Input: dimensioned drawing with shaded views. Units: mm. Origin: part minimum x, y, z. A direction names the side the tool comes from. Coordinates: 2 decimals unless noted, no trailing zeros. Loops run counter-clockwise (first coordinate to the right, second up) from the corner with the lowest first, then second, coordinate; pieces in that order, holes last.
Item 1: Contact query for flat-ended pins moving along their axis: P1, Ø4, axis at x = 198.5, y = 184.5, coming from the +Z side; P2, Ø6, axis at y = 120, z = 552.5, coming from the -X side; P3, Ø6, axis at y = 65, z = 941.5, coming from the +X side. Output: stop coordinate, or through.
Item 2: Section C-C on z = 563.5. Return loops of the section in (x, y), and give its area (3 significant figures).
Item 3: Section B-B on x = 825.5. Return loops of the section in (y, z).
Item 4: Pull-direction query (Z, two-part tool) for the marked faces 4, 5 and 6; classes: released by +Z, released by -Z, zero draft, split by the parting line, or undercut.
Item 5: Section A-A on y = 143. Return loops of the section in (x, z) (1 decimal), and give its area (3 significant figures).
Item 6: Reachability of the marked faces 1, 2 and 3 from +Z, -Z, +X, -X, +Y, -Y: full face, straight path, thin tool, end or side. Return the list, or none.
Item 7: Section D-D on x = 416. Return loops of the section in (y, z).
Item 8: Ray query, line 1 along Z through (x, y) = (825, 111); line 2 along X through (y, z) = (43.5, 372); line 3 along Z through (x, y) = (148, 86). Return the intervals inside material, ascending.
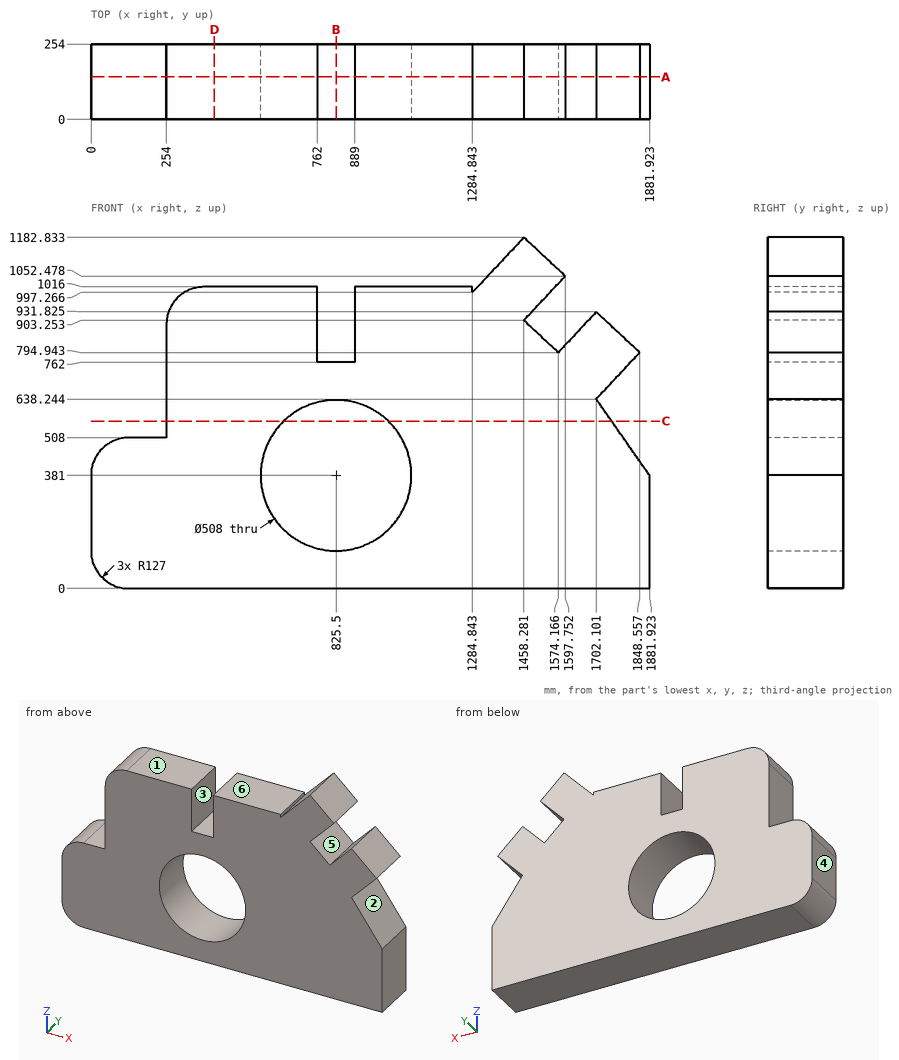
Results found:
1. P1: stops at z = 508
1. P2: stops at x = 254
1. P3: stops at x = 1496.83
2. outline: (254, 0) - (648.84, 0) - (648.84, 254) - (254, 254) - close; (1002.16, 0) - (1754.35, 0) - (1754.35, 254) - (1002.16, 254) - close
2. area: 291,000 mm2
3. outline: (0, 0) - (254, 0) - (254, 127) - (0, 127) - close; (0, 635) - (254, 635) - (254, 762) - (0, 762) - close
4. face 4: zero draft
4. face 5: undercut
4. face 6: released by +Z
5. outline: (0, 127) arc R127 ccw to (127, 0) - (1881.9, 0) - (1881.9, 381) - (1702.1, 638.2) - (1848.6, 794.9) - (1702.1, 931.8) - (1574.2, 794.9) - (1458.3, 903.3) - (1597.8, 1052.5) - (1458.3, 1182.8) - (1284.8, 997.3) - (1284.8, 1016) - (889, 1016) - (889, 762) - (762, 762) - (762, 1016) - (381, 1016) arc R127 ccw to (254, 889) - (254, 508) - (127, 508) arc R127 ccw to (0, 381) - close; hole circle Ø508 at (825.5, 381)
5. area: 1,460,000 mm2
6. face 1: +Z, -X, +Y, -Y
6. face 2: +X, +Y, -Y
6. face 3: +Z, +Y, -Y
7. outline: (0, 0) - (254, 0) - (254, 1016) - (0, 1016) - close
8. line 1: z = 0 to 127, 635 to 762
8. line 2: x = 0 to 571.66, 1079.34 to 1881.92
8. line 3: z = 0 to 508
